Read the model definition and answer for the solid it produces. Units are mm, in the model's axes. Face numbers are marked on the shaded views. Give positions to 0.01 mm unless a question says otherwise; leave off trailing zeros. Order: outer loops, then holes, each group sorted by start corner. A loop starts at its lowest first (then second) coordinate and runs counter-clockwise, first axis right, second up.
Item 1: Given pin 1 Ø6 at (y, z) = (-36, 7) entering from -X; pin 2 Ø1.5 at (x, z) = (-6, 67.5) entering from +Y; pin 3 Ø5 at (x, y) = (-17, -6.5) entering from -Z, each flat-ended and moving along its own axis, determine where each tip first touches the part or whether it passes through.
Item 2: A cutting plane is placed at D-D (z = 47). Write down the section's boundary in (x, y), plus the area to 3 significant figures.
Item 3: The mould has two halves that part along Z. Classify the marked faces 1, 2, 3 and 4: +Z half, -Z half, draft (parallel to the pull), parting line (faces both ways), or undercut.
Item 4: Find the intervals of material crossed by line 1 along Z through (x, y) = (-8.5, -24); line 2 along Y through (x, z) = (8.5, 84); line 3 along Z through (x, y) = (-1, -35), in increasing order.
Item 5: A cutting plane is placed at C-C (x = 0). Write down the section's boundary in (y, z).
Item 6: A cutting plane is placed at B-B (y = -24). Write down the section's boundary in (x, z).
Item 7: A cutting plane is placed at A-A (x = -66). Write down the section's boundary in (y, z).
from build123d import *

# Parameters (mm, degrees)
F0_R          = 3.81
F1_DEPTH      = 38.1
F3_DEPTH      = 2.54
F4_R          = 15.875
F5_DEPTH      = 57.912
F7_DEPTH      = 40.64
F7_DEPTH_BACK = 30.988
F9_DEPTH      = 140.716
F11_DEPTH     = 2.54
F12_R         = 25.4
F13_R         = 3.175
F14_DEPTH     = 25.4


with BuildPart() as f1:
    # F0 (on Front) → F1 (new body)
    with BuildSketch(Plane.XZ):
        Circle(F0_R)
    extrude(amount=F1_DEPTH)

    # F2 (on face) → F3 (join)
    with BuildSketch(Plane.XZ.offset(38.1)):
        with BuildLine():
            ThreePointArc((-12.7, 0), (0, -12.7), (12.7, 0))
            ThreePointArc((12.7, 0), (0, 12.7), (-12.7, 0))
        make_face()
        with BuildLine():
            ThreePointArc((-12.7, 0), (0, 12.7), (12.7, 0))
            Line((12.7, 0), (12.7, 101.6))
            Line((12.7, 101.6), (-63.5, 101.6))
            Line((-63.5, 101.6), (-63.5, 76.2))
            Line((-63.5, 76.2), (-12.7, 0))
        make_face()
    extrude(amount=F3_DEPTH)

    # F4 (on face) → F5 (join)
    with BuildSketch(Plane.XY.offset(101.6)):
        with Locations((-66.675, -28.575)):
            Circle(F4_R)
    extrude(amount=-F5_DEPTH)

    # F6 (on face) → F7 (cut, two sides)
    with BuildSketch(Plane.XZ.offset(40.64)) as f7_sk:
        with BuildLine():
            Line((-44.4512212261, -6.503643468), (-12.7, 0))
            Line((-12.7, 0), (-56.3574712261, 65.4862068392))
            ThreePointArc((-56.3574712261, 65.4862068392), (-73.8011886318, 82.898697178), (-84.6138894558, 105.0473675132))
            Line((-84.6138894558, 105.0473675132), (-88.3945673704, 14.1553971916))
            Line((-88.3945673704, 14.1553971916), (-44.4512212261, -6.503643468))
        make_face()
    extrude(amount=-F7_DEPTH, mode=Mode.SUBTRACT)
    extrude(f7_sk.sketch, amount=F7_DEPTH_BACK, mode=Mode.SUBTRACT)

    # F8 (on face) → F9 (cut)
    with BuildSketch(Plane.YZ.offset(12.7)):
        Polygon((-6.1655906029, 4.6855383553), (-6.1655906029, 63.5), (-6.1655906029, 99.06), (-38.1, 99.06), (-38.1, 4.6855383553), align=None)
    extrude(amount=-F9_DEPTH, mode=Mode.SUBTRACT)

    # F10 (on face) → F11 (join)
    with BuildSketch(Plane.XY.offset(101.6)):
        with BuildLine():
            Line((-53.975, -38.1), (12.7, -38.1))
            Line((12.7, -38.1), (12.7, 0))
            Line((12.7, 0), (-3.81, 0))
            Line((-3.81, 0), (-68.9945726443, -12.8703762303))
            ThreePointArc((-68.9945726443, -12.8703762303), (-53.0341863545, -20.4544194735), (-53.975, -38.1))
        make_face()
    extrude(amount=-F11_DEPTH)

    # F12
    f12_edges = [f1.edges().sort_by_distance(p)[0] for p in [
        (-56.357471, -40.64, 83.543103),
    ]]
    fillet(f12_edges, radius=F12_R)

    # F13 (on face) → F14 (cut)
    with BuildSketch(Plane.XY.offset(101.6)):
        with Locations((-66.675, -28.575)):
            Circle(F13_R)
    extrude(amount=-F14_DEPTH, mode=Mode.SUBTRACT)


solid = f1.part
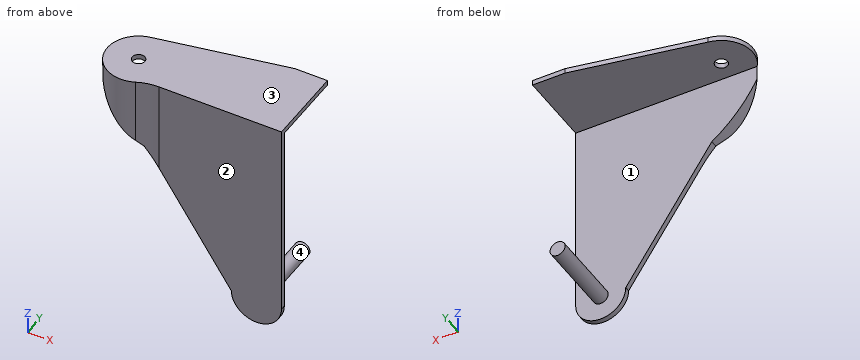
Response values:
1. pin 1: stops at x = -18.79
1. pin 2: stops at y = -38.1
1. pin 3: stops at z = 99.06
2. outline: (-44.03, -40.64) - (12.7, -40.64) - (12.7, -38.1) - (-44.03, -38.1) - close
2. area: 144 mm2
3. face 1: undercut
3. face 2: draft
3. face 3: +Z half
3. face 4: undercut
4. line 1: z = 99.06 to 101.6
4. line 2: y = -40.64 to -38.1
4. line 3: z = -3.68 to 3.68, 99.06 to 101.6
5. outline: (-40.64, -12.7) - (-38.1, -12.7) - (-38.1, -3.81) - (0, -3.81) - (0, 3.81) - (-38.1, 3.81) - (-38.1, 99.06) - (0, 99.06) - (0, 101.6) - (-40.64, 101.6) - close
6. outline: (-81.88, 99.06) - (12.7, 99.06) - (12.7, 101.6) - (-81.88, 101.6) - close; circle Ø7.62 at (0, 0)
7. outline: (-44.44, 73.66) - (-38.1, 73.66) - (-38.1, 99.06) - (-31.68, 99.06) - (-31.68, 101.6) - (-44.44, 101.6) - close; (-25.47, 99.06) - (-12.28, 99.06) - (-12.28, 101.6) - (-25.47, 101.6) - close
